from build123d import *

# Parameters (mm, degrees)
BOSS_EXTRUDE1_DEPTH = 10
SKETCH3_R           = 7.535275438
CUT_EXTRUDE10_DEPTH = 10


with BuildPart() as part:
    # Sketch1 → Boss-Extrude1 (new body)
    with BuildSketch(Plane(origin=(0, 0, 0), x_dir=(1, 0, 0), z_dir=(0, 1, 0))):
        with BuildLine():
            Line((73.562221188, 48.852459016), (-106.437778812, 48.852459016))
            ThreePointArc((-106.437778812, 48.852459016), (-113.508846624, 45.923526828), (-116.437778812, 38.852459016))
            Line((-116.437778812, 38.852459016), (-116.437778812, -41.147540984))
            ThreePointArc((-116.437778812, -41.147540984), (-113.508846624, -48.218608795), (-106.437778812, -51.147540984))
            Line((-106.437778812, -51.147540984), (73.562221188, -51.147540984))
            ThreePointArc((73.562221188, -51.147540984), (80.633289, -48.218608795), (83.562221188, -41.147540984))
            Line((83.562221188, -41.147540984), (83.562221188, 38.852459016))
            ThreePointArc((83.562221188, 38.852459016), (80.633289, 45.923526828), (73.562221188, 48.852459016))
        make_face()
    extrude(amount=BOSS_EXTRUDE1_DEPTH)

    # Sketch3 → Cut-Extrude10 (cut)
    with BuildSketch(Plane(origin=(0, 0, 0), x_dir=(1, 0, 0), z_dir=(0, 1, 0))):
        with Locations((48.215632939, 37.678714221)):
            Circle(SKETCH3_R)
        with Locations((19.480783272, 37.678714221)):
            Circle(SKETCH3_R)
        with Locations((48.215632939, -31.079676053)):
            Circle(SKETCH3_R)
        with Locations((19.480783272, -31.079676053)):
            Circle(SKETCH3_R)
        with Locations((-76.302048951, 0)):
            Circle(SKETCH3_R)
        with Locations((19.480783272, -8.606914665)):
            Circle(SKETCH3_R)
        with Locations((48.215632939, -8.606914665)):
            Circle(SKETCH3_R)
        with Locations((19.480783272, 15.338793391)):
            Circle(SKETCH3_R)
        with Locations((50.268122201, 15.338793391)):
            Circle(SKETCH3_R)
    extrude(amount=CUT_EXTRUDE10_DEPTH, mode=Mode.SUBTRACT)


solid = part.part
Geometry: final body of the model. Coordinates: model frame, mm. Coordinates: 2 decimals unless noted, no trailing zeros. Order: outer loops, then holes, each group sorted by start corner. A loop starts at its lowest first (then second) coordinate and runs counter-clockwise, first axis right, second up.
(1) Material intervals for probe 1 along X at (y, z) = (7.25, 0); probe 2 along Z at (x, y) = (25.5, 9.25); probe 3 along X at (y, z) = (0.5, 9), sorted ascending.
(2) Section query B-B (z = -19.5). Return the cut outline in (x, y).
(3) Section query C-C (y = 8.5). State how many separate pieces and enclosed holes the cut face has, plus the area to 3 significant figures.
(4) Section query A-A (x = 25). Return the cut outline in (y, z).
(5) Draft query along X for faces 1 (the face through (-18, 0, 0)), 2 (the face through (-113.586, 4.93, 48.14)), 3 (the face through (51.693, 4.93, 37.765)), 4 (the face through (80.711, 4.93, -45.845)). Return one class per face: pulls with the +X half, pulls with the -X half, needs draft (parallel to the pull), parting line crosses it, or undercut.
Solution:
1. probe 1: x = -116.44 to -83.84, -68.77 to 83.56
1. probe 2: z = -48.85 to -42.21, -33.15 to -19.87, -10.81 to 4.07, 13.14 to 26.55, 35.61 to 51.15
1. probe 3: x = -116.44 to 11.96, 27.01 to 40.69, 55.74 to 83.56
2. outline: (-116.44, 0) - (13.2, 0) - (13.2, 10) - (-116.44, 10) - close; (25.76, 0) - (43.99, 0) - (43.99, 10) - (25.76, 10) - close; (56.55, 0) - (83.56, 0) - (83.56, 10) - (56.55, 10) - close
3. separate pieces: 1
3. enclosed holes: 9
3. area: 18,300 mm2
4. outline: (0, -48.85) - (10, -48.85) - (10, -42.81) - (0, -42.81) - close; (0, -32.55) - (10, -32.55) - (10, -20.47) - (0, -20.47) - close; (0, -10.21) - (10, -10.21) - (10, 3.48) - (0, 3.48) - close; (0, 13.74) - (10, 13.74) - (10, 25.95) - (0, 25.95) - close; (0, 36.21) - (10, 36.21) - (10, 51.15) - (0, 51.15) - close
5. face 1: needs draft
5. face 2: pulls with the -X half
5. face 3: undercut
5. face 4: pulls with the +X half
